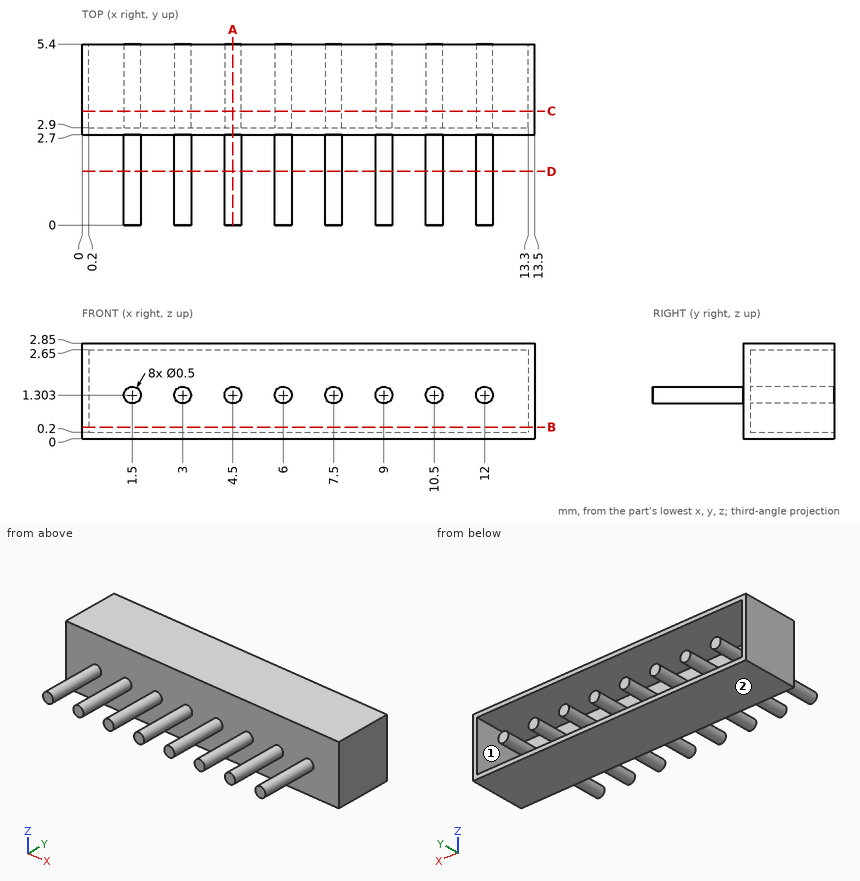
Geometry check sheet. Reference: drawing and pictorial views, mm from the part's lowest x, y, z. A direction names the side the tool comes from. Round coordinates to 2 decimals unless told otherwise and drop trailing zeros. Loops run counter-clockwise (first coordinate to the right, second up) from the corner with the lowest first, then second, coordinate; pieces in that order, holes last. Notation, with made-up numbers: (-7, -9) - (37, -9) arc R30 ccw to (37, 25) - close; hole circle Ø2 at (88.25, 57). An arc over 180 degrees is marked (long way). Answer as CSV lines item,"result".
(1) Material ranges on line 1 along Z through (x, y) = (12, 3.05); line 2 along Z through (x, y) = (0.75, 3.8); line 3 along X through (y, z) = (3.5, 2.15), recorded low to high.
Output values:
line 1,"z = 0 to 0.2, 1.05 to 1.55, 2.65 to 2.85"
line 2,"z = 0 to 0.2, 2.65 to 2.85"
line 3,"x = 0 to 0.2, 13.3 to 13.5"
(2) Cross-section at A-A, the plane x = 4.5. Enter the section's corners in (y, z).
Output values:
outline,"(0, 1.05) - (2.7, 1.05) - (2.7, 0) - (5.4, 0) - (5.4, 0.2) - (2.9, 0.2) - (2.9, 1.05) - (5.4, 1.05) - (5.4, 1.55) - (2.9, 1.55) - (2.9, 2.65) - (5.4, 2.65) - (5.4, 2.85) - (2.7, 2.85) - (2.7, 1.55) - (0, 1.55) - close"
(3) Set-up check for the marked faces 1 and 2: record each of +Z, -Z, +X, -X, +Y, -Y from which the full face is reachable in a straight line by a thin tool's end or side.
Output values:
face 1,"+Y"
face 2,"-Z, +X, -X, +Y, -Y"
(4) Cross-section at C-C, the plane y = 3.4. Give the number of separate pieces and of enclosed holes in the cut face.
Output values:
separate pieces,"9"
enclosed holes,"1"
(5) Cross-section at B-B, the plane z = 0.35. Enter the section's corners in (x, y).
Output values:
outline,"(0, 2.7) - (13.5, 2.7) - (13.5, 5.4) - (13.3, 5.4) - (13.3, 2.9) - (0.2, 2.9) - (0.2, 5.4) - (0, 5.4) - close"
(6) Cross-section at D-D, the plane y = 1.6. Enter the section's corners in (x, z).
Output values:
outline,"circle Ø0.5 at (1.5, 1.3); circle Ø0.5 at (3, 1.3); circle Ø0.5 at (4.5, 1.3); circle Ø0.5 at (6, 1.3); circle Ø0.5 at (7.5, 1.3); circle Ø0.5 at (9, 1.3); circle Ø0.5 at (10.5, 1.3); circle Ø0.5 at (12, 1.3)"
